```python
from build123d import *

# Parameters (mm, degrees)
F1_DEPTH = 15
F2_R     = 4
F3_DEPTH = 25


with BuildPart() as f1:
    # F0 (on Front) → F1 (new body, symmetric)
    with BuildSketch(Plane.XZ):
        Polygon((-50, 5), (-50, 0), (-30, 0), (-19.739396, 28.190779), (-24.437859, 29.900879), (-33.501038, 5), align=None)
    extrude(amount=F1_DEPTH, both=True)

    # F2 (on face) → F3 (cut)
    with BuildSketch(Plane.XY.offset(5)):
        with Locations((-42, 0)):
            Circle(F2_R)
    extrude(amount=-F3_DEPTH, mode=Mode.SUBTRACT)


solid = f1.part
```
For this review, take the finished solid that the model builds, in its own axes (mm). A direction names the side the tool comes from. Give positions to 0.01 mm unless a question says otherwise; leave off trailing zeros. Order: outer loops, then holes, each group sorted by start corner. A loop starts at its lowest first (then second) coordinate and runs counter-clockwise, first axis right, second up.
1) For faces 1 (the face through (-31.6, 15, 9.5)), 2 (the face through (-40, -4, 5)), list the 3-axis set-ups (+Z, -Z, +X, -X, +Y, -Y) from which the entire face can be reached by the end or side of a thin tool; tool diameter is ignored.
2) Take a section at A-A (y = 0). Give the boundary of the cut face in (x, z), then the cut area to 3 significant figures.
3) Take a section at D-D (y = 13). Give the boundary of the cut face in (x, z).
4) The part is to be moulded in two halves that separate along X. For faces 3 (the face through (-28.906, -0.21, 17.625)), 4 (the face through (-24.94, -0.21, 13.9)), 5 (the face through (-45.2, -2.4, 2.5)), 6 (the face through (-40, -4, 0)), say which applies: released by +X, released by -X, zero draft, split by the parting line, or undercut.
5) Insertion check: pin 1 (3 mm diameter, centred on y = -10.5, z = 14, fed in from +X); pin 2 (4 mm diameter, centred on y = 10.5, z = 9.5, fed in from +X); pin 3 (8 mm diameter, centred on y = 8.5, z = 15, fed in from -X). Each pin has a flat end and moves straight along its axis. Give the tip position at first contact, or say it passes through.
6) Take a section at C-C (z = 4.25). Give the boundary of the cut face in (x, y), then the cut area to 3 significant figures.
7) Wall thickness on line 1 (Y direction, x = -42, z = 3.4); line 2 (Z direction, x = -42.5, y = -6.25); line 3 (X direction, y = -12.25, z = 19.75): over which ranges is each line inside the solid? List them lowest first.
8) Take a section at B-B (x = -42). Give the boundary of the cut face in (y, z).
Derived:
1. face 1: +Z, -Z, +X, -X, +Y
1. face 2: +Z, -X, +Y, -Y
2. outline: (-50, 0) - (-46, 0) - (-46, 5) - (-50, 5) - close; (-38, 0) - (-30, 0) - (-19.74, 28.19) - (-24.44, 29.9) - (-33.5, 5) - (-38, 5) - close
2. area: 192 mm2
3. outline: (-50, 0) - (-30, 0) - (-19.74, 28.19) - (-24.44, 29.9) - (-33.5, 5) - (-50, 5) - close
4. face 3: released by -X
4. face 4: released by +X
4. face 5: undercut
4. face 6: zero draft
5. pin 1: stops at x = -24.36
5. pin 2: stops at x = -25.81
5. pin 3: stops at x = -31.32
6. outline: (-50, -15) - (-28.45, -15) - (-28.45, 15) - (-50, 15) - close; hole circle Ø8 at (-42, 0)
6. area: 596 mm2
7. line 1: y = -15 to -4, 4 to 15
7. line 2: z = 0 to 5
7. line 3: x = -28.13 to -22.81
8. outline: (-15, 0) - (-4, 0) - (-4, 5) - (-15, 5) - close; (4, 0) - (15, 0) - (15, 5) - (4, 5) - close
